Study the drawing (mm; zero at the part's minimum x, y, z) and answer. Coordinates: 2 decimals unless noted, no trailing zeros. Loops run counter-clockwise (first coordinate to the right, second up) from the corner with the lowest first, then second, coordinate; pieces in that order, holes last.
Q1. Flat-ended cylindrical pins translate along their axes: P1, Ø5, axis at x = 104.87, z = 37.25, coming from the -Y side; P2, Ø3, axis at x = 85, y = 1.5, coming from the -Z side; P3, Ø3, axis at x = 62, z = 12.5, coming from the +Y side; P4, Ø1.5, axis at x = 86, y = 1, coming from the -Z side (1 decimal). Find the tip coordinate at first contact, or state that the pin passes through.
Q2. Section B-B (x = 62) is taken. Give the vertices of the cut face in (y, z), then the cut area to 3 significant figures.
Q3. Straight lines are drawn through the part: line 1 (X direction, y = 2.1, z = 86.75) (1 decimal); line 2 (X direction, y = 1.65, z = 62); line 3 (X direction, y = 2.05, z = 37.25) (1 decimal). For each, find the intervals that lie inside material, in ascending order.
Q4. Section C-C (x = 76) is taken. Give the vertices of the cut face in (y, z).
Q5. Section D-D (y = 1.35) is taken. Give the vertices of the cut face in (x, z), then the cut area to 3 significant figures.
Q6. Section A-A (z = 62) is taken. Give the vertices of the cut face in (x, y).
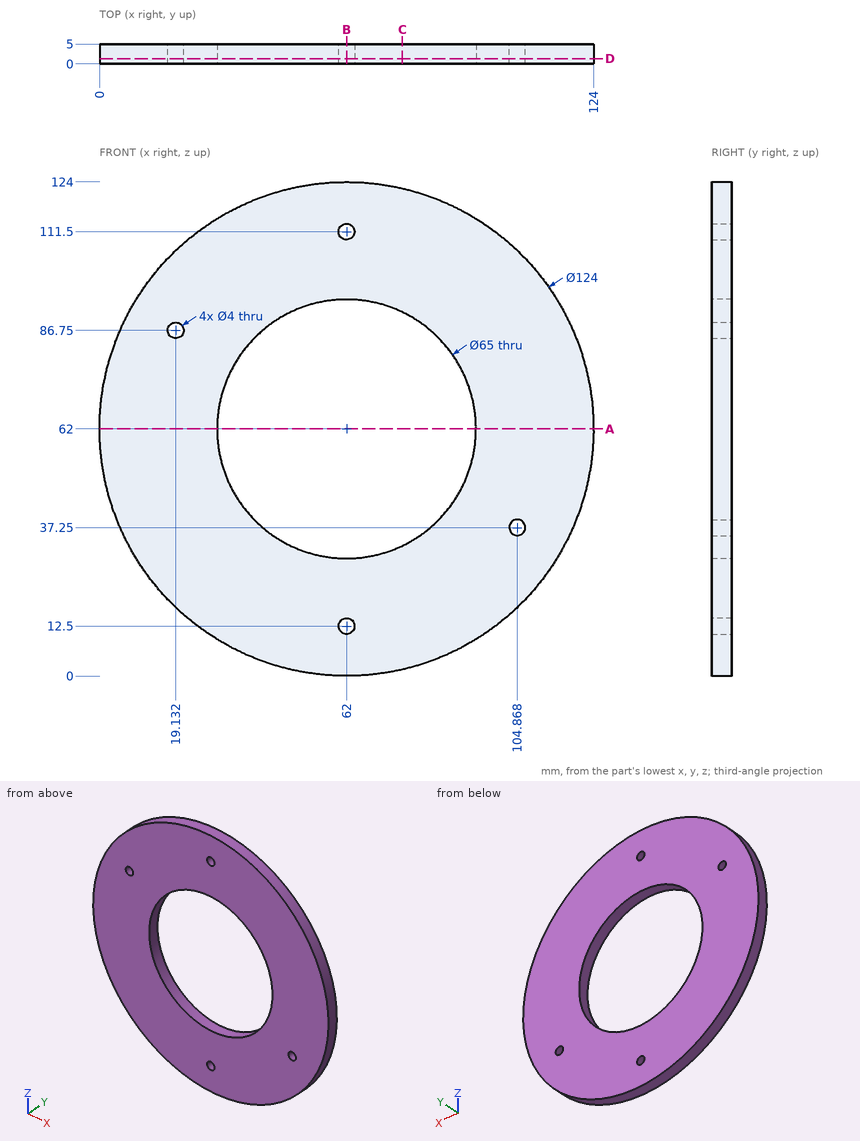
Numbers:
1. P1: stops at y = 0
1. P2: stops at z = 3.85
1. P3: passes through
1. P4: stops at z = 4.5
2. outline: (0, 0) - (5, 0) - (5, 10.5) - (0, 10.5) - close; (0, 14.5) - (5, 14.5) - (5, 29.5) - (0, 29.5) - close; (0, 94.5) - (5, 94.5) - (5, 109.5) - (0, 109.5) - close; (0, 113.5) - (5, 113.5) - (5, 124) - (0, 124) - close
2. area: 255 mm2
3. line 1: x = 5.2 to 17.1, 21.1 to 40.9, 83.1 to 118.8
3. line 2: x = 0 to 29.5, 94.5 to 124
3. line 3: x = 5.2 to 40.9, 83.1 to 102.9, 106.9 to 118.8
4. outline: (0, 1.6) - (5, 1.6) - (5, 32.67) - (0, 32.67) - close; (0, 91.33) - (5, 91.33) - (5, 122.4) - (0, 122.4) - close
5. outline: circle Ø124 at (62, 62); hole circle Ø4 at (19.13, 86.75); hole circle Ø65 at (62, 62); hole circle Ø4 at (62, 12.5); hole circle Ø4 at (62, 111.5); hole circle Ø4 at (104.87, 37.25)
5. area: 8,710 mm2
6. outline: (0, 0) - (29.5, 0) - (29.5, 5) - (0, 5) - close; (94.5, 0) - (124, 0) - (124, 5) - (94.5, 5) - close
